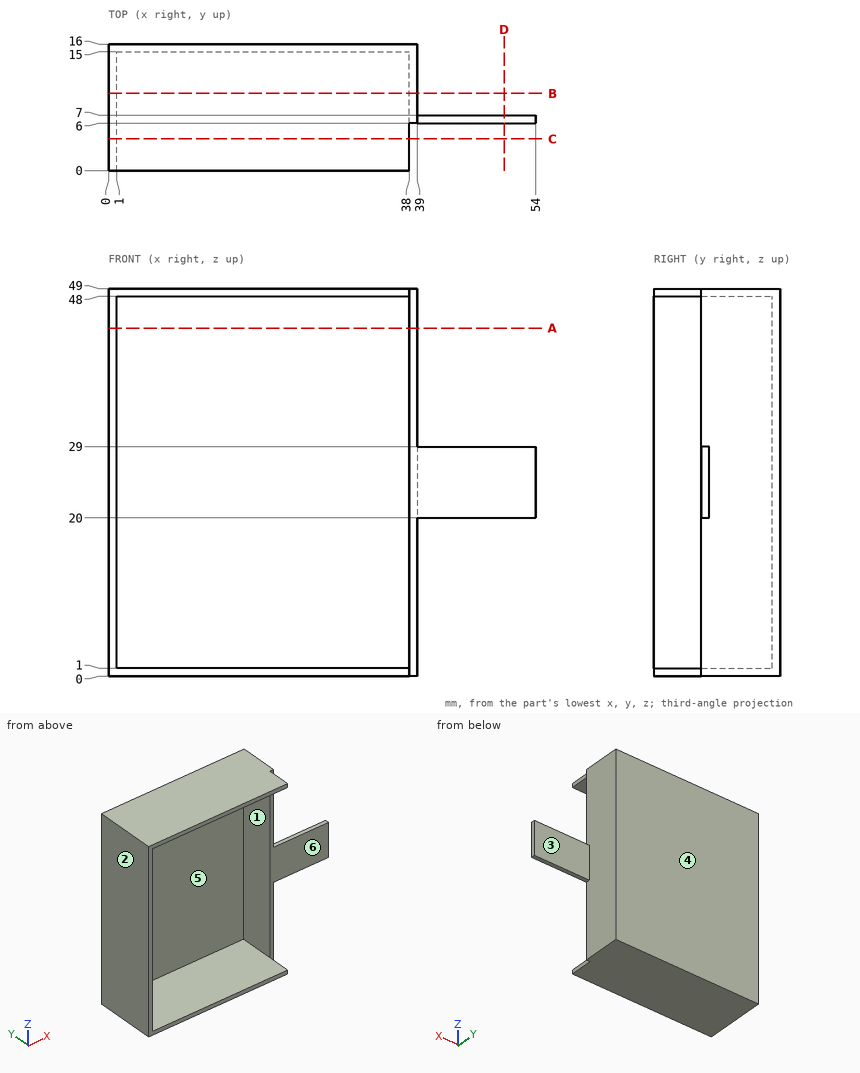
Geometry: see drawing. Coordinates: mm, zero at the bounding-box minimum. A direction names the side the tool comes from. Coordinates: 2 decimals unless noted, no trailing zeros. Loops run counter-clockwise (first coordinate to the right, second up) from the corner with the lowest first, then second, coordinate; pieces in that order, holes last. Notation, with made-up numbers: M -6,13 L 3,13 A17 ccw 3,25 Z; hole C -17,50.25 d4. An arc over 180 degrees is marked long. Put each result on its own line as item: value. Start each with the question number.
1) Contact query for flat-ended pins moving along their axis: pin 1 Ø0.5 at (x, y) = (49, 6.5) entering from +Z; pin 2 Ø1.1 at (x, y) = (45, 6.5) entering from -Z; pin 3 Ø12 at (x, z) = (44, 28) entering from +Y; pin 4 Ø1.1 at (y, z) = (4, 0.5) entering from +X. Output: stop coordinate, or through.
2) Cut plane A-A on z = 44. Return the cut outline in (x, y).
3) Cut plane D-D on x = 50. Return the cut outline in (y, z).
4) Cut plane B-B on y = 9.75. Return the cut outline in (x, z).
5) Cut plane C-C on y = 4. Return the cut outline in (x, z), then the cut area to 3 significant figures.
6) Reachability of the marked faces 4, 5 and 6 from +Z, -Z, +X, -X, +Y, -Y: full face, straight path, thin tool, end or side. Return the list, or none.
7) Ray query, L1, parallel to X at y = 11.25, z = 46; L2, parallel to Z at x = 14, y = 2.75; L3, parallel to Y at x = 24, z = 13. Return the intervals inside material, ascending. Write a range as from..to.
8) Pull-direction query (X, two-part tool) for the marked faces 1, 2 and 3; classes: pulls with the +X half, pulls with the -X half, needs draft (parallel to the pull), parting line crosses it, or undercut.
The answers:
1. pin 1: stops at z = 29
1. pin 2: stops at z = 20
1. pin 3: stops at y = 16
1. pin 4: stops at x = 38
2. outline: M 0,0 L 1,0 L 1,15 L 38,15 L 38,6 L 39,6 L 39,16 L 0,16 Z
3. outline: M 6,20 L 7,20 L 7,29 L 6,29 Z
4. outline: M 0,0 L 39,0 L 39,49 L 0,49 Z; hole M 1,1 L 38,1 L 38,48 L 1,48 Z
5. outline: M 0,0 L 38,0 L 38,1 L 1,1 L 1,48 L 38,48 L 38,49 L 0,49 Z
5. area: 123 mm²
6. face 4: +Z, -Z, +X, -X, +Y
6. face 5: -Y
6. face 6: +Z, -Z, +X, -Y
7. L1: x = 0..1, 38..39
7. L2: z = 0..1, 48..49
7. L3: y = 15..16
8. face 1: undercut
8. face 2: pulls with the -X half
8. face 3: needs draft
